Drawing for the job (mm, zero at the part's lowest x, y, z). A direction names the side the tool comes from. Round coordinates to 2 decimals unless told otherwise and drop trailing zeros. Loops run counter-clockwise (first coordinate to the right, second up) from the corner with the lowest first, then second, coordinate; pieces in that order, holes last. Notation, with made-up numbers: M 51,34 L 92,34 A17 ccw 92,47 Z; hole C 10,47.5 d5. An arc over 180 degrees is marked long. Answer in a Markdown table with one row per item.
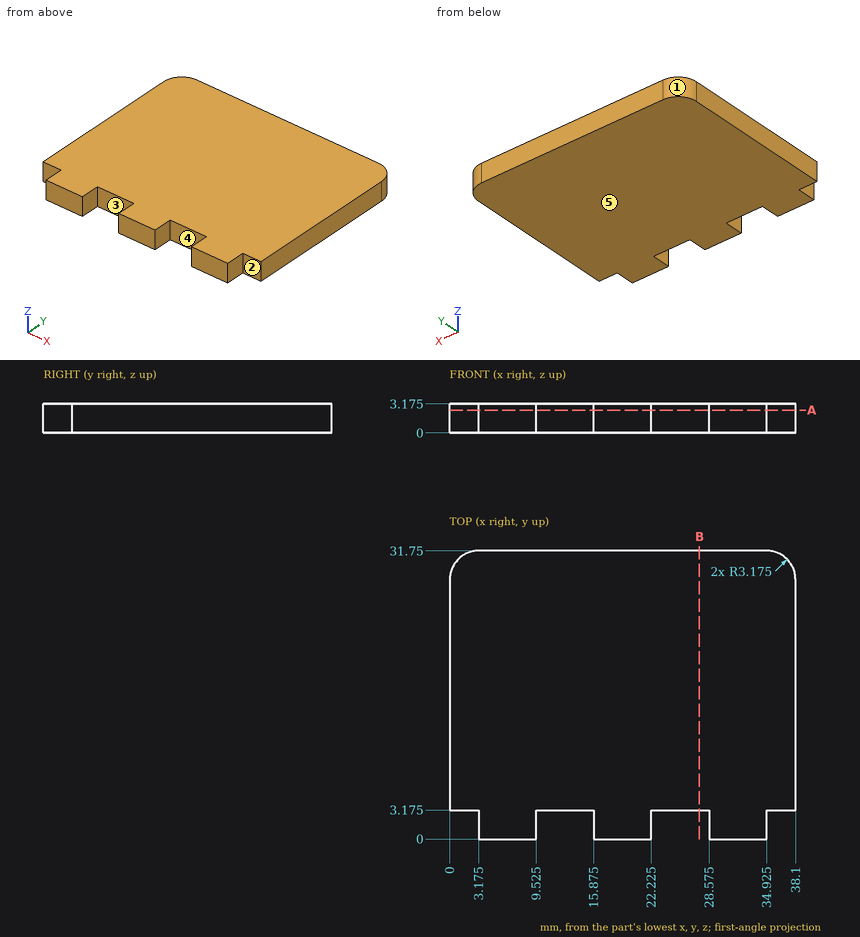
1. Wall check: probe 1 along X at (y, z) = (2, 0.5) (3 decimals); probe 2 along Y at (x, z) = (22.5, 2.4) (3 decimals); probe 3 along Y at (x, z) = (2, 2) (3 decimals). Give the ranges that are in metal, low to high.
Verdict:
| item | result |
|---|---|
| probe 1 | x = 3.175 to 9.525, 15.875 to 22.225, 28.575 to 34.925 |
| probe 2 | y = 3.175 to 31.75 |
| probe 3 | y = 3.175 to 31.525 |
2. Pin check, flat tips, straight feed: pin 1 (1 mm diameter, centred on y = 2.5, z = 1.5, fed in from +X) (3 decimals); pin 2 (1 mm diameter, centred on x = 12.5, z = 2, fed in from -Y) (3 decimals); pin 3 (1 mm diameter, centred on y = 2.5, z = 2, fed in from -X) (3 decimals). Stop position of each tip, or through.
Verdict:
| item | result |
|---|---|
| pin 1 | stops at x = 34.925 |
| pin 2 | stops at y = 3.175 |
| pin 3 | stops at x = 3.175 |
3. Tool access for the marked faces 4 and 5: list every direction of +Z, -Z, +X, -X, +Y, -Y with a clear straight run to the whole face (end or side of a thin tool).
Verdict:
| item | result |
|---|---|
| face 4 | +Z, -Z, -Y |
| face 5 | -Z, +X, -X, +Y, -Y |
4. Saw through at A-A (z = 2.5). Write the cut outline in (x, y) (3 decimals).
Verdict:
| item | result |
|---|---|
| outline | M 0,3.175 L 3.175,3.175 L 3.175,0 L 9.525,0 L 9.525,3.175 L 15.875,3.175 L 15.875,0 L 22.225,0 L 22.225,3.175 L 28.575,3.175 L 28.575,0 L 34.925,0 L 34.925,3.175 L 38.1,3.175 L 38.1,28.575 A3.175 ccw 34.925,31.75 L 3.175,31.75 A3.175 ccw 0,28.575 Z |
5. Saw through at B-B (x = 27.5). Write the cut outline in (y, z) (3 decimals), and give its area (3 significant figures).
Verdict:
| item | result |
|---|---|
| outline | M 3.175,0 L 31.75,0 L 31.75,3.175 L 3.175,3.175 Z |
| area | 90.7 mm² |
6. Mould opens along X. For the marked faces 1, 2 and 3 say: +X half, -X half, draft (parallel to the pull), parting line (faces both ways), or undercut.
Verdict:
| item | result |
|---|---|
| face 1 | -X half |
| face 2 | draft |
| face 3 | undercut |
